Source: CAD feature listing. Evaluate the final solid. Frame: model axes, mm. Face numbers are marked on the shaded views. A direction names the side the tool comes from. Coordinates: 2 decimals unless noted, no trailing zeros. Write each loop counter-clockwise with the first axis right and the second up, starting at its lowest first coordinate (ties: lowest second). Pieces come first, ordered by that corner, then holes. Notation, with made-up numbers: (44.25, 4) - (88.25, 4) arc R14 ccw to (88.25, 16) - close; hole circle Ø1 at (22, -27.5). An arc over 180 degrees is marked (long way). One line per item, written item: value.
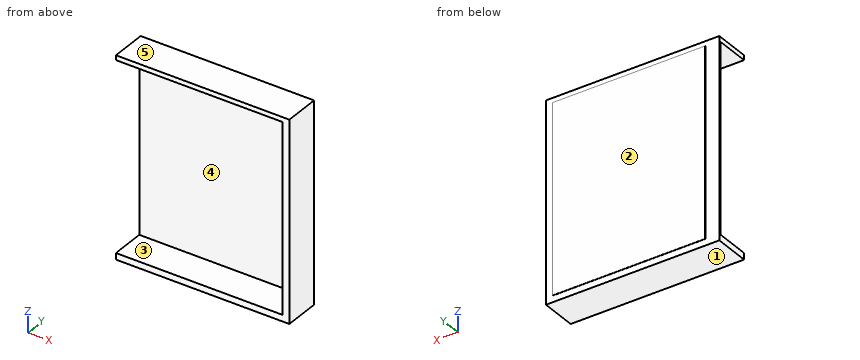
Autodesk Inventor part; units mm, degrees
ref_plane "YZ Plane" through (0, 0, 0) normal (1, 0, 0) x (0, 1, 0)
ref_plane "XZ Plane" through (0, 0, 0) normal (0, 1, 0) x (-1, 0, 0)
ref_plane "XY Plane" through (0, 0, 0) normal (0, 0, 1) x (1, 0, 0)
sketch "Sketch1" plane through (0, 0, 0) normal (0, 1, 0) x (-1, 0, 0)
  line L0 (14.2304, 19.7891) -> (-36.5696, 19.7891)
  line L1 (-36.5696, 19.7891) -> (-36.5696, -38.6309)
  line L2 (-36.5696, -38.6309) -> (14.2304, -38.6309)
  line L3 (14.2304, -38.6309) -> (14.2304, 19.7891)
  point P0 (0, 0)
  dimension "d0" = 50.8
  dimension "d1" = 58.42
extrude "Extrusion1" add sketch "Sketch1" along normal blind 10.4902
sketch "Sketch2" plane through (0, 0, 0) normal (0, -1, 0) x (1, 0, 0)
  line L0 (34.5988, 18.3949) -> (-14.5151, 18.3949)
  line L1 (-14.5151, 18.3949) -> (-14.5151, -36.7441)
  line L2 (-14.5151, -36.7441) -> (34.5988, -36.7441)
  line L3 (34.5988, -36.7441) -> (34.5988, 18.3949)
  point P0 (0, 0)
extrude "Extrusion2" cut sketch "Sketch2" against normal blind 9.906
sketch "Sketch3" plane through (0, 10.4902, 0) normal (0, 1, 0) x (1, 0, 0)
  line L0 (34.5988, 36.7441) -> (-14.2304, 36.7441)
  line L1 (-14.2304, -18.3949) -> (34.5988, -18.3949)
  line L2 (34.5988, 36.7441) -> (-10.1332, 36.7441)
  line L3 (-10.1332, 36.7441) -> (-10.1332, -18.3949)
  line L4 (-10.1332, -18.3949) -> (34.5988, -18.3949)
  line L5 (34.5988, -18.3949) -> (34.5988, 36.7441)
  point P0 (0, 0)
extrude "Extrusion3" add sketch "Sketch3" along normal blind 0.0762
properties part number "glasscover" material "Glass"
1) Material intervals for line 1 (Z direction, x = 4, y = 3.5); line 2 (X direction, y = 6.5, z = -24.5); line 3 (Y direction, x = 25, z = -13), sorted ascending.
Values found:
line 1: -38.63 to -36.74, 18.39 to 19.79
line 2: 34.6 to 36.57
line 3: 9.91 to 10.57
2) Reachability of the marked faces 4 and 5 from +Z, -Z, +X, -X, +Y, -Y: full face, straight path, thin tool, end or side. Return the list, or none.
Values found:
face 4: -X, -Y
face 5: +Z, +X, -X, +Y, -Y
3) Draft query along Z for the marked faces 1, 2 and 3. Return one class per face: released by +Z, released by -Z, zero draft, split by the parting line, or undercut.
Values found:
face 1: released by -Z
face 2: zero draft
face 3: undercut
4) Section query B-B on x = 6.5. Output: boundary loops of the cut face in (y, z), then the cut area to 3 significant figures.
Values found:
outline: (0, -38.63) - (10.49, -38.63) - (10.49, -36.74) - (10.57, -36.74) - (10.57, 18.39) - (10.49, 18.39) - (10.49, 19.79) - (0, 19.79) - (0, 18.39) - (9.91, 18.39) - (9.91, -36.74) - (0, -36.74) - close
area: 70.8 mm2
5) Section query A-A on y = 8.75. Output: boundary loops of the cut face in (x, z).
Values found:
outline: (-14.23, -38.63) - (36.57, -38.63) - (36.57, 19.79) - (-14.23, 19.79) - (-14.23, 18.39) - (34.6, 18.39) - (34.6, -36.74) - (-14.23, -36.74) - close
6) Section query C-C on z = -22.5. Output: boundary loops of the cut face in (x, y).
Values found:
outline: (-14.23, 9.91) - (34.6, 9.91) - (34.6, 0) - (36.57, 0) - (36.57, 10.49) - (34.6, 10.49) - (34.6, 10.57) - (-10.13, 10.57) - (-10.13, 10.49) - (-14.23, 10.49) - close
7) Contact query for flat-ended pins moving along their axis: P1, Ø5, axis at y = 4, z = -16.5, coming from the -X side; P2, Ø1, axis at x = 24, z = -30.5, coming from the -Y side. Output: stop coordinate, or through.
Values found:
P1: x = 34.6
P2: y = 9.91
